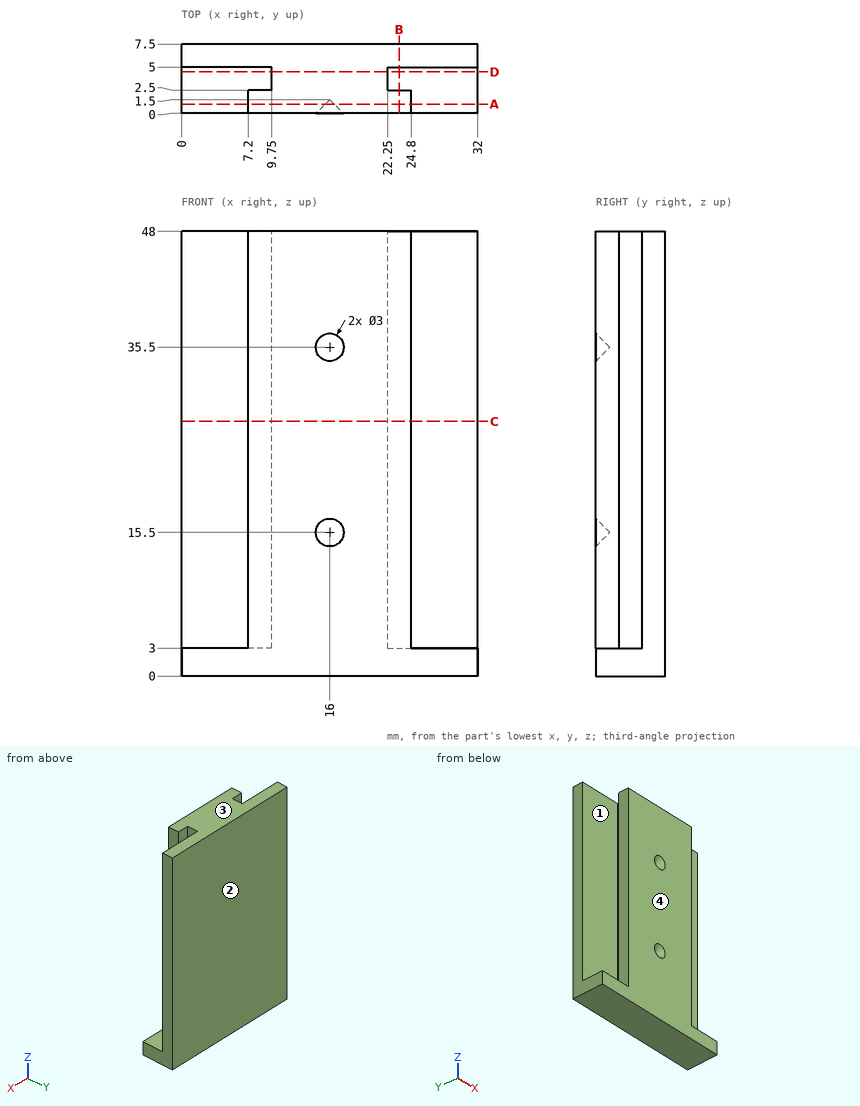
Can you work these out from the drawing? Everything is in mm from the part's minimum corner. Give positions to 0.01 mm unless a question says otherwise; leave off trailing zeros. Loops run counter-clockwise (first coordinate to the right, second up) from the corner with the lowest first, then second, coordinate; pieces in that order, holes last. Notation, with made-up numbers: M 46.5,-7.5 L 61.5,-7.5 A8 ccw 61.5,-0.5 Z; hole C 89,-34.75 d1. An arc over 180 degrees is marked long. Put each result on its own line as item: value. Start each with the question number.
(1) I want a section at B-B on x = 23.5. Please give me the cut outline in (y, z).
(2) If we mould it in two halves opening along Y, with no side actions, what happens to the marked faces 1, 2, 3 and 4? For each: +Y half, -Y half, draft (parallel to the pull), parting line (faces both ways), or undercut.
(3) I want a section at A-A on y = 1. Please give me the cut outline in (x, z), then the cut area to 3 significant figures.
(4) Will these pins go through, and if not, where does the flat tip stop? pin 1 Ø1 at (y, z) = (6.5, 15) entering from -X; pin 2 Ø0.8 at (y, z) = (1.5, 22.5) entering from +X; pin 3 Ø1.2 at (y, z) = (3.5, 34) entering from -X; pin 4 Ø3 at (x, z) = (28, 26) entering from -Y.
(5) I want a section at D-D on y = 4.5. Please give me the cut outline in (x, z).
(6) I want a section at C-C on z = 27.5. Please give me the cut outline in (x, y).
(7) I need wall thicknesses on line 1 along X through (y, z) = (1.5, 14); line 2 along Y through (x, z) = (4, 43); line 3 along X through (y, z) = (3.75, 20.5). Which ranges of each line are inside material? Lowest first, please. Write a range as [from, to].
Answer block:
1. outline: M 0,0 L 7.5,0 L 7.5,48 L 5,48 L 5,3 L 2.5,3 L 2.5,48 L 0,48 Z
2. face 1: undercut
2. face 2: +Y half
2. face 3: draft
2. face 4: -Y half
3. outline: M 0,0 L 32,0 L 32,3 L 24.8,3 L 24.8,48 L 7.2,48 L 7.2,3 L 0,3 Z; hole C 16,15.5 d1; hole C 16,35.5 d1
3. area: 886 mm^2
4. pin 1: x = 0
4. pin 2: x = 24.8
4. pin 3: x = 9.75
4. pin 4: y = 5
5. outline: M 0,0 L 32,0 L 32,3 L 22.25,3 L 22.25,48 L 9.75,48 L 9.75,3 L 0,3 Z
6. outline: M 0,5 L 9.75,5 L 9.75,2.5 L 7.2,2.5 L 7.2,0 L 24.8,0 L 24.8,2.5 L 22.25,2.5 L 22.25,5 L 32,5 L 32,7.5 L 0,7.5 Z
7. line 1: [7.2, 24.8]
7. line 2: [5, 7.5]
7. line 3: [9.75, 22.25]
